Autodesk Inventor part; units mm, degrees
ref_plane "MSC_PF1" through (0, 0, 0) normal (1, 0, 0) x (0, 1, 0)
ref_plane "MSC_PT1" through (3.9, 0, -0.58) normal (0, 0, -1) x (-1, 0, 0)
ref_plane "YZ Plane" through (0, 0, 0) normal (1, 0, 0) x (0, 1, 0)
sketch "Esquisse2" plane through (0, 0, 0) normal (0, 1, 0) x (-1, 0, 0)
  line L0 (0, -10) -> (-2, -10)
  line L1 (0, 0) -> (0, -10)
  line L2 (-3.9, 0) -> (0, 0)
  line L3 (-3.9, -0.58) -> (-3.9, 0)
  line L4 (-2, -2.48) -> (-3.9, -0.58)
  line L5 (-2, -10) -> (-2, -2.48)
  line L6 (0, 0) -> (0, -10)
  dimension "d2" = 45
  dimension "d4" = 2
  dimension "d6" = 3.9
  dimension "d8" = 2.48
  dimension "d10" = 10
revolve "Révolution1" add sketch "Esquisse2" angle 360 about axis through (0, 0, 0) along (0, 0, -1)
fillet "Congé1" radius 0.35 1 edges at (-2, 0, -2.48)
chamfer "Chanfrein1" distance 0.35 angle 45 1 edges at (-2, 0, -10)
sketch "Esquisse4" plane through (0, 0, 0) normal (0, 0, 1) x (1, 0, 0)
  circle A0 centre (0, 0) radius 3.9
  circle A1 centre (0, 0) radius 1.25 construction
  line L0 (-1.25, -0.7217) -> (-1.25, 0.7217)
  line L1 (-1.25, 0.7217) -> (0, 1.4434)
  line L2 (0, 1.4434) -> (1.25, 0.7217)
  line L3 (1.25, 0.7217) -> (1.25, -0.7217)
  line L4 (1.25, -0.7217) -> (0, -1.4434)
  line L5 (0, -1.4434) -> (-1.25, -0.7217)
  dimension "d27" = 2.5
extrude "Extrusion1" cut sketch "Esquisse4" against normal blind 1.5 contours L0 L1 L2 L3 L4 L5
sketch "Esquisse5" plane through (0, 0, 0) normal (0, 0, 1) x (1, 0, 0)
  circle A0 centre (0, 0) radius 3.9
  circle A1 centre (0, 0) radius 1.2625
  dimension "d38" = 2.525
extrude "Extrusion2" cut sketch "Esquisse5" against normal blind 1.5 contours A1
thread "Filetage1"
ref_plane "MSC_PF1" through (0, 0, 0) normal (1, 0, 0) x (0, 1, 0)
ref_plane "MSC_PT1" through (3.9, 0, -0.58) normal (0, 0, -1) x (-1, 0, 0)
equation "\"d4\" = 0.5 * NND"
equation "\"d6\" = 0.5 * ParA"
equation "\"d8\" = ParH"
equation "\"d10\" = NLG"
equation "\"d27\" = ParJ"
equation "\"d39\" = Tt"
equation "\"d24\" = Rr"
equation "\"d25\" = 0.5 * PTC"
equation "\"d26\" = 0.5 * PTC"
equation "\"d28\" = Tt"
equation "\"d31\" = Lt"
equation "\"d38\" = 1.01 * ParJ"
equation "\"NND\" = 4"
equation "\"NLG\" = 10"
equation "\"PTC\" = 0.7"
equation "\"ParA\" = 7.8"
equation "\"ParH\" = 2.48"
equation "\"ParJ\" = 2.5"
equation "\"Tt\" = 1.5"
equation "\"Rr\" = 0.35"
equation "\"msp_e\" = 0.288675 * ParJ"
equation "\"Lt\" = 6.12"
equation "\"THREADDIA\" = NND"
properties part number "ASME/ANSI B18.3.5M - M4x10(2)" material "Acier, doux"
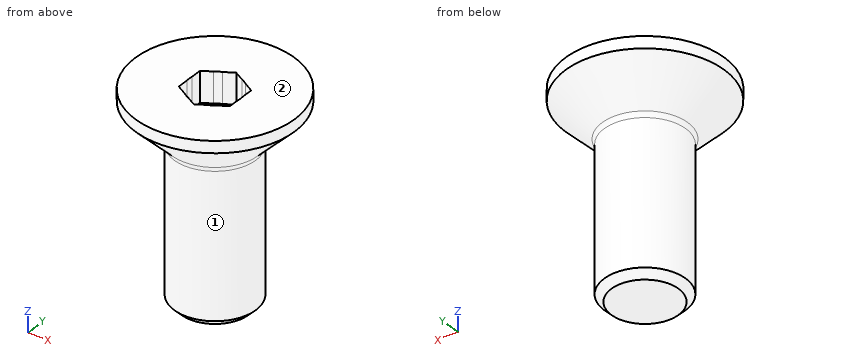
Input: part model. Units: mm. Frame: model coordinates. Face numbers are marked on the shaded views. A direction names the side the tool comes from. Give positions to 0.01 mm unless a question says otherwise; leave off trailing zeros. Order: outer loops, then holes, each group sorted by start corner. A loop starts at its lowest first (then second) coordinate and runs counter-clockwise, first axis right, second up.
Q1. Contact query for flat-ended pins moving along their axis: pin 1 Ø1.3 at (x, y) = (0, 0) entering from +Z; pin 2 Ø0.6 at (y, z) = (-0.5, -0.5) entering from -X; pin 3 Ø0.6 at (y, z) = (0.5, -1) entering from -X. Output: stop coordinate, or through.
Checked values:
pin 1: stops at z = -1.5
pin 2: stops at x = -3.89
pin 3: stops at x = -3.75
Q2. Section B-B on z = -8.5. Output: boundary loops of the cut face in (x, y).
Checked values:
outline: circle Ø4 at (0, 0)
Q3. Ray query, probe 1 along Z at (x, y) = (3.25, -1.25); probe 2 along X at (y, z) = (0.25, -4.25); probe 3 along Y at (x, z) = (1.75, -0.5). Return the intervals inside material, ascending.
Checked values:
probe 1: z = -1 to 0
probe 2: x = -1.98 to 1.98
probe 3: y = -3.49 to 3.49
Q4. Set-up query: the marked faces 1 and 2. Return all of +Z, -Z, +X, -X, +Y, -Y with unobstructed straight access to the full face (end or side cutting, diameter ignored); none if empty.
Checked values:
face 1: -Z
face 2: +Z, +X, -X, +Y, -Y
